Here's how the part is built. I have some questions about the finished solid (model axes, mm). A direction names the side the tool comes from. Round coordinates to 2 decimals unless told otherwise and drop trailing zeros. Loops run counter-clockwise (first coordinate to the right, second up) from the corner with the lowest first, then second, coordinate; pieces in that order, holes last. Notation, with made-up numbers: (-32, 48.25) -> (12, 48.25) arc R23 ccw to (12, 66.25) -> close; hole circle Ø5 at (86.5, 78.25). An arc over 180 degrees is marked (long way). Use one line per item in the form item = value. Start each with the question number.
Item 1: If I drill on L1, parallel to X at y = 162.5, z = 2.2; L2, parallel to Y at x = -108.5, z = 9; L3, parallel to Y at x = -73, z = 9.25, over which ranges is the centre line in solid material (lowest first)? Write a range as [from, to].
Item 2: If we section it at B-B (y = 62.5): State how many separate pieces and enclosed holes the cut face has, then the cut area to 3 significant figures.
Item 3: Thinking about a two-plate mould opening in Y: for faces 4 (the face through (-113.195, 87.729, 6.549)), 5 (the face through (-90.34, 84.79, 14.93)), which applies, released by +Y, released by -Y, zero draft, split by the parting line, or undercut?
Item 4: If we section it at A-A (z = 13): Write out the boundary of the cut face in (x, y).
Item 5: I'm going to push flat-ended pins straight in: pin 1 Ø11.5 at (x, y) = (-31, 14.5) entering from +Z; pin 2 Ø5 at (x, y) = (-60.5, 93) entering from -Z; pin 3 Ø7.5 at (x, y) = (-8, 187.5) entering from +Z. Where does each tip first touch, or does it pass through?
Item 6: For faces 1 (the face through (-63.427, 91.335, 2.465)), 2 (the face through (-36.2, 187.6, 1.5)), 3 (the face through (-113.195, 12.729, 6.549)), which set-ups out of +Z, -Z, +X, -X, +Y, -Y let a thin tool reach every point of the face, with its end or its side?
```python
from build123d import *

# Parameters (mm, degrees)
SKETCH_1_W          = 141
SKETCH_1_H          = 200
EXTRUDE_1_DEPTH     = 10
SKETCH_5_R          = 5
SKETCH_5_R_2        = 2.75
CUT_EXTRUDE_5_DEPTH = 245.91018762
SKETCH_6_R          = 5
CUT_EXTRUDE_6_DEPTH = 5
SKETCH_7_R          = 25
EXTRUDE_2_DEPTH     = 10
SKETCH_8_R          = 2.75
SKETCH_8_R_2        = 5
CUT_EXTRUDE_7_DEPTH = 10
SKETCH_9_R          = 3.2
CUT_EXTRUDE_8_DEPTH = 50
SKETCH_10_R         = 5.2
CUT_EXTRUDE_9_DEPTH = 7


with BuildPart() as part:
    # 스케치1 → 보스-돌출1 (new body)
    with BuildSketch(Plane.XY):
        with Locations((-70.5, 100)):
            Rectangle(SKETCH_1_W, SKETCH_1_H)
    extrude(amount=EXTRUDE_1_DEPTH)

    # 스케치5 → 컷-돌출5 (cut, through all)
    with BuildSketch(Plane.XY):
        with Locations((-70.5, 100)):
            Circle(SKETCH_5_R)
        with Locations((-70.5, 113.5)):
            Circle(SKETCH_5_R_2)
        with Locations((-58.808657049, 106.75)):
            Circle(SKETCH_5_R_2)
        with Locations((-58.808657049, 93.25)):
            Circle(SKETCH_5_R_2)
        with Locations((-70.5, 86.5)):
            Circle(SKETCH_5_R_2)
        with Locations((-82.191342951, 93.25)):
            Circle(SKETCH_5_R_2)
        with Locations((-82.191342951, 106.75)):
            Circle(SKETCH_5_R_2)
    extrude(amount=CUT_EXTRUDE_5_DEPTH, mode=Mode.SUBTRACT)

    # 스케치6 → 컷-돌출6 (cut)
    with BuildSketch(Plane(origin=(0, 0, 0), x_dir=(-1, 0, 0), z_dir=(0, 0, -1))):
        with Locations((70.5, 113.5)):
            Circle(SKETCH_6_R)
        with Locations((82.191342951, 106.75)):
            Circle(SKETCH_6_R)
        with Locations((82.191342951, 93.25)):
            Circle(SKETCH_6_R)
        with Locations((70.5, 86.5)):
            Circle(SKETCH_6_R)
        with Locations((58.808657049, 93.25)):
            Circle(SKETCH_6_R)
        with Locations((58.808657049, 106.75)):
            Circle(SKETCH_6_R)
    extrude(amount=-CUT_EXTRUDE_6_DEPTH, mode=Mode.SUBTRACT)

    # 스케치7 → 보스-돌출2 (add)
    with BuildSketch(Plane.XY.offset(10)):
        with Locations((-70.5, 100)):
            Circle(SKETCH_7_R)
    extrude(amount=EXTRUDE_2_DEPTH)

    # 스케치8 → 컷-돌출7 (cut)
    with BuildSketch(Plane(origin=(0, 0, 10), x_dir=(-1, 0, 0), z_dir=(0, 0, -1))):
        with Locations((82.191342951, 106.75)):
            Circle(SKETCH_8_R)
        with Locations((82.191342951, 93.25)):
            Circle(SKETCH_8_R)
        with Locations((70.5, 86.5)):
            Circle(SKETCH_8_R)
        with Locations((58.808657049, 93.25)):
            Circle(SKETCH_8_R)
        with Locations((58.808657049, 106.75)):
            Circle(SKETCH_8_R)
        with Locations((70.5, 113.5)):
            Circle(SKETCH_8_R)
        with Locations((70.5, 100)):
            Circle(SKETCH_8_R_2)
    extrude(amount=-CUT_EXTRUDE_7_DEPTH, mode=Mode.SUBTRACT)

    # 스케치9 → 컷-돌출8 (cut)
    with BuildSketch(Plane.XY.offset(10)):
        with Locations((-8, 187.5)):
            Circle(SKETCH_9_R)
        with Locations((-8, 12.5)):
            Circle(SKETCH_9_R)
        with Locations((-133, 187.5)):
            Circle(SKETCH_9_R)
        with Locations((-133, 12.5)):
            Circle(SKETCH_9_R)
        with Locations((-33, 187.5)):
            Circle(SKETCH_9_R)
        with Locations((-58, 187.5)):
            Circle(SKETCH_9_R)
        with Locations((-83, 187.5)):
            Circle(SKETCH_9_R)
        with Locations((-108, 187.5)):
            Circle(SKETCH_9_R)
        with Locations((-8, 162.5)):
            Circle(SKETCH_9_R)
        with Locations((-8, 137.5)):
            Circle(SKETCH_9_R)
        with Locations((-8, 112.5)):
            Circle(SKETCH_9_R)
        with Locations((-8, 87.5)):
            Circle(SKETCH_9_R)
        with Locations((-8, 62.5)):
            Circle(SKETCH_9_R)
        with Locations((-8, 37.5)):
            Circle(SKETCH_9_R)
        with Locations((-133, 162.5)):
            Circle(SKETCH_9_R)
        with Locations((-133, 137.5)):
            Circle(SKETCH_9_R)
        with Locations((-133, 112.5)):
            Circle(SKETCH_9_R)
        with Locations((-133, 87.5)):
            Circle(SKETCH_9_R)
        with Locations((-133, 62.5)):
            Circle(SKETCH_9_R)
        with Locations((-133, 37.5)):
            Circle(SKETCH_9_R)
        with Locations((-108, 12.5)):
            Circle(SKETCH_9_R)
        with Locations((-83, 12.5)):
            Circle(SKETCH_9_R)
        with Locations((-58, 12.5)):
            Circle(SKETCH_9_R)
        with Locations((-33, 12.5)):
            Circle(SKETCH_9_R)
        with Locations((-33, 112.5)):
            Circle(SKETCH_9_R)
        with Locations((-33, 87.5)):
            Circle(SKETCH_9_R)
        with Locations((-108, 112.5)):
            Circle(SKETCH_9_R)
        with Locations((-108, 87.5)):
            Circle(SKETCH_9_R)
        with Locations((-58, 137.5)):
            Circle(SKETCH_9_R)
        with Locations((-83, 137.5)):
            Circle(SKETCH_9_R)
        with Locations((-58, 62.5)):
            Circle(SKETCH_9_R)
        with Locations((-83, 62.5)):
            Circle(SKETCH_9_R)
    extrude(amount=-CUT_EXTRUDE_8_DEPTH, mode=Mode.SUBTRACT)

    # 스케치10 → 컷-돌출9 (cut)
    with BuildSketch(Plane.XY.offset(10)):
        with Locations((-8, 187.5)):
            Circle(SKETCH_10_R)
        with Locations((-33, 187.5)):
            Circle(SKETCH_10_R)
        with Locations((-58, 187.5)):
            Circle(SKETCH_10_R)
        with Locations((-83, 187.5)):
            Circle(SKETCH_10_R)
        with Locations((-108, 187.5)):
            Circle(SKETCH_10_R)
        with Locations((-133, 187.5)):
            Circle(SKETCH_10_R)
        with Locations((-8, 162.5)):
            Circle(SKETCH_10_R)
        with Locations((-8, 137.5)):
            Circle(SKETCH_10_R)
        with Locations((-8, 112.5)):
            Circle(SKETCH_10_R)
        with Locations((-8, 87.5)):
            Circle(SKETCH_10_R)
        with Locations((-8, 62.5)):
            Circle(SKETCH_10_R)
        with Locations((-8, 37.5)):
            Circle(SKETCH_10_R)
        with Locations((-8, 12.5)):
            Circle(SKETCH_10_R)
        with Locations((-33, 12.5)):
            Circle(SKETCH_10_R)
        with Locations((-58, 12.5)):
            Circle(SKETCH_10_R)
        with Locations((-83, 12.5)):
            Circle(SKETCH_10_R)
        with Locations((-108, 12.5)):
            Circle(SKETCH_10_R)
        with Locations((-133, 12.5)):
            Circle(SKETCH_10_R)
        with Locations((-133, 162.5)):
            Circle(SKETCH_10_R)
        with Locations((-133, 137.5)):
            Circle(SKETCH_10_R)
        with Locations((-133, 112.5)):
            Circle(SKETCH_10_R)
        with Locations((-133, 87.5)):
            Circle(SKETCH_10_R)
        with Locations((-133, 62.5)):
            Circle(SKETCH_10_R)
        with Locations((-133, 37.5)):
            Circle(SKETCH_10_R)
        with Locations((-33, 112.5)):
            Circle(SKETCH_10_R)
        with Locations((-33, 87.5)):
            Circle(SKETCH_10_R)
        with Locations((-58, 62.5)):
            Circle(SKETCH_10_R)
        with Locations((-83, 62.5)):
            Circle(SKETCH_10_R)
        with Locations((-108, 87.5)):
            Circle(SKETCH_10_R)
        with Locations((-108, 112.5)):
            Circle(SKETCH_10_R)
        with Locations((-83, 137.5)):
            Circle(SKETCH_10_R)
        with Locations((-58, 137.5)):
            Circle(SKETCH_10_R)
    extrude(amount=-CUT_EXTRUDE_9_DEPTH, mode=Mode.SUBTRACT)


solid = part.part
```
Values found:
q1.L1 = [-141, -136.2], [-129.8, -11.2], [-4.8, 0]
q1.L2 = [0, 7.32], [17.68, 82.32], [92.68, 107.32], [117.68, 182.32], [192.68, 200]
q1.L3 = [0, 85.35], [87.65, 95.67], [104.33, 112.35], [114.65, 200]
q2.separate_pieces = 5
q2.enclosed_holes = 0
q2.area = 1,040 mm2
q3.face_4 = undercut
q3.face_5 = split by the parting line
q4.outline = circle Ø50 at (-70.5, 100); hole circle Ø5.5 at (-82.19, 93.25); hole circle Ø5.5 at (-82.19, 106.75); hole circle Ø10 at (-70.5, 100); hole circle Ø5.5 at (-70.5, 86.5); hole circle Ø5.5 at (-70.5, 113.5); hole circle Ø5.5 at (-58.81, 93.25); hole circle Ø5.5 at (-58.81, 106.75)
q5.pin_1 = 10
q5.pin_2 = 5
q5.pin_3 = 3
q6.face_1 = -Z
q6.face_2 = +Z, -Z
q6.face_3 = +Z
